Check sheet for the modelled part. Datum: model origin and axes. Units: mm. A direction names the side the tool comes from. Round coordinates to 2 decimals unless told otherwise and drop trailing zeros. Write each loop counter-clockwise with the first axis right and the second up, starting at its lowest first coordinate (ties: lowest second). Pieces come first, ordered by that corner, then holes. Notation, with made-up numbers: (5.5, 30) -> (22.5, 30) arc R28 ccw to (22.5, 66) -> close; hole circle Ø3 at (9, -10.75). An arc over 180 degrees is marked (long way). One line per item, written item: value.
from build123d import *

# Parameters (mm, degrees)
ESQUISSE1_W              = 175
ESQUISSE1_H              = 277
BOSS_EXTRU_2_DEPTH       = 190
ESQUISSE2_W              = 80
ESQUISSE2_H              = 80
ENL_V_MAT_EXTRU_2_DEPTH  = 15
ESQUISSE6_R              = 6.5
BOSS_EXTRU_4_DEPTH       = 15
CHANFREIN2_SIZE          = 1
ENL_V_START              = -10
ESQUISSE12_OUTSIDE_W     = 252.75
ESQUISSE12_OUTSIDE_H     = 354.75
ESQUISSE12_OUTSIDE_W_2   = 155
ESQUISSE12_OUTSIDE_H_2   = 257
ENL_V_MAT_EXTRU_5_DEPTH  = 155
CHANFREIN5_SIZE          = 10
CONG_1_R                 = 5
ENL_V_MAT_EXTRU_10_REACH = 326.86
ESQUISSE13_R             = 2.5
CHANFREIN8_SIZE          = 5
CONG_3_R                 = 10
ESQUISSE14_R             = 10
ESQUISSE14_R_2           = 9
ENL_V_MAT_EXTRU_11_DEPTH = 1
ESQUISSE15_W             = 4
ESQUISSE15_H             = 10
ENL_V_MAT_EXTRU_12_DEPTH = 1


with BuildPart() as part:
    # Esquisse1 → Boss.-Extru.2 (new body)
    with BuildSketch(Plane.XY):
        with Locations((87.5, 138.5)):
            Rectangle(ESQUISSE1_W, ESQUISSE1_H)
    extrude(amount=BOSS_EXTRU_2_DEPTH)

    # Esquisse2 → Enlèv. mat.-Extru.2 (cut)
    with BuildSketch(Plane.XY.offset(190)):
        with Locations((135, 40)):
            Rectangle(ESQUISSE2_W, ESQUISSE2_H)
        with Locations((135, 237)):
            Rectangle(ESQUISSE2_W, ESQUISSE2_H)
    extrude(amount=-ENL_V_MAT_EXTRU_2_DEPTH, mode=Mode.SUBTRACT)

    # Esquisse6 → Boss.-Extru.4 (add)
    with BuildSketch(Plane.XY.offset(175)):
        with Locations((135, 40)):
            Circle(ESQUISSE6_R)
        with Locations(Location((135, 237, 0), (0, 0, 180))):
            Circle(ESQUISSE6_R)
    extrude(amount=BOSS_EXTRU_4_DEPTH)

    # Chanfrein2
    chanfrein2_edges = [part.edges().sort_by_distance(p)[0] for p in [
        (128.5, 40, 190),
        (141.5, 237, 190),
    ]]
    chamfer(chanfrein2_edges, length=CHANFREIN2_SIZE)

    # Esquisse12 outside → Enlèv. mat.-Extru.5 (cut)
    with BuildSketch(Plane(origin=(0, 0, 0), x_dir=(-1, 0, 0), z_dir=(0, 0, -1)).offset(ENL_V_START)):
        with Locations((-87.5, 138.5)):
            Rectangle(ESQUISSE12_OUTSIDE_W, ESQUISSE12_OUTSIDE_H)
        with Locations((-87.5, 138.5)):
            Rectangle(ESQUISSE12_OUTSIDE_W_2, ESQUISSE12_OUTSIDE_H_2, mode=Mode.SUBTRACT)
    extrude(amount=-ENL_V_MAT_EXTRU_5_DEPTH, mode=Mode.SUBTRACT)

    # Chanfrein5
    chanfrein5_edges = [part.edges().sort_by_distance(p)[0] for p in [
        (165, 138.5, 10),
        (87.5, 267, 10),
        (10, 138.5, 10),
        (87.5, 10, 10),
    ]]
    chamfer(chanfrein5_edges, length=CHANFREIN5_SIZE - 0.0001)  # a hair under: the kernel refuses the full size

    # Congé1
    cong_1_edges = [part.edges().sort_by_distance(p)[0] for p in [
        (175, 138.5, 190),
        (135, 80, 190),
        (95, 40, 190),
        (47.5, 277, 190),
        (95, 237, 190),
        (135, 197, 190),
        (0, 138.5, 190),
        (47.5, 0, 190),
    ]]
    fillet(cong_1_edges, radius=CONG_1_R)

    # Esquisse13 → Enlèv. mat.-Extru.10 (cut, up to next)
    with BuildSketch(Plane.XZ.offset(-80), mode=Mode.PRIVATE) as enl_v_mat_extru_10_sk1:
        with Locations((100, 180)):
            Circle(ESQUISSE13_R)
    enl_v_mat_extru_10_tool1 = extrude(enl_v_mat_extru_10_sk1.sketch, amount=-ENL_V_MAT_EXTRU_10_REACH, mode=Mode.PRIVATE) & part.part
    # Esquisse13 → Enlèv. mat.-Extru.10 (cut, up to next)
    with BuildSketch(Plane.XZ.offset(-80), mode=Mode.PRIVATE) as enl_v_mat_extru_10_sk2:
        with BuildLine():
            Line((145, 175), (175, 175))
            Line((175, 175), (175, 190))
            Line((175, 190), (135, 190))
            Line((135, 190), (135, 185))
            ThreePointArc((135, 185), (137.928932188, 177.928932188), (145, 175))
        make_face()
    enl_v_mat_extru_10_tool2 = extrude(enl_v_mat_extru_10_sk2.sketch, amount=-ENL_V_MAT_EXTRU_10_REACH, mode=Mode.PRIVATE) & part.part
    add(enl_v_mat_extru_10_tool1.solids().sort_by_distance((100, 80, 180))[0], mode=Mode.SUBTRACT)
    add(enl_v_mat_extru_10_tool2.solids().sort_by_distance((155.659019, 80, 182.695347))[0], mode=Mode.SUBTRACT)

    # Chanfrein8
    chanfrein8_edges = [part.edges().sort_by_distance(p)[0] for p in [
        (135, 81.464466094, 188.535533906),
        (137.928932188, 80, 177.928932188),
        (137.928932188, 197, 177.928932188),
        (135, 195.535533906, 188.535533906),
        (135, 138.5, 190),
    ]]
    chamfer(chanfrein8_edges, length=CHANFREIN8_SIZE - 0.0001)  # a hair under: the kernel refuses the full size

    # Congé3
    cong_3_edges = [part.edges().sort_by_distance(p)[0] for p in [
        (87.5, 267, 165),
        (165, 138.5, 165),
        (87.5, 10, 165),
        (10, 138.5, 165),
    ]]
    fillet(cong_3_edges, radius=CONG_3_R - 0.0001)  # a hair under: the kernel refuses the full size

    # Esquisse14 → Enlèv. mat.-Extru.11 (cut)
    # profile 1 of 2: a face of its own
    with BuildSketch(Plane.XY.offset(175)):
        with Locations((158.25, 40)):
            Circle(ESQUISSE14_R)
        with Locations((158.25, 40)):
            Circle(ESQUISSE14_R_2, mode=Mode.SUBTRACT)
    # profile 2 of 2: a face of its own
    with BuildSketch(Plane.XY.offset(175)):
        with Locations(Location((158.25, 237, 0), (0, 0, 180))):
            Circle(ESQUISSE14_R)
        with Locations(Location((158.25, 237, 0), (0, 0, 180))):
            Circle(ESQUISSE14_R_2, mode=Mode.SUBTRACT)
    extrude(amount=-ENL_V_MAT_EXTRU_11_DEPTH, mode=Mode.SUBTRACT)

    # Esquisse15 → Enlèv. mat.-Extru.12 (cut)
    with BuildSketch(Plane.XY.offset(175)):
        with Locations((158.25, 40)):
            Rectangle(ESQUISSE15_W, ESQUISSE15_H)
        Polygon((156.583333333, 235.333333333), (153.25, 235.333333333), (153.25, 238.666666667), (156.583333333, 238.666666667), (156.583333333, 242), (159.916666667, 242), (159.916666667, 238.666666667), (163.25, 238.666666667), (163.25, 235.333333333), (159.916666667, 235.333333333), (159.916666667, 232), (156.583333333, 232), align=None)
    extrude(amount=-ENL_V_MAT_EXTRU_12_DEPTH, mode=Mode.SUBTRACT)


solid = part.part
Item 1: Release check for a two-part mould opening along X. For faces 4 (the cylindrical face through (165.39, 242.48, 174.51)), 5 (the flat face through (86, 140, 0)), 6 (the cylindrical face through (6.99, 140.44, 162.15)) record: pulls with the +X half, pulls with the -X half, needs draft (parallel to the pull), parting line crosses it, or undercut.
Result set:
face 4: undercut
face 5: needs draft
face 6: pulls with the -X half
Item 2: Material ranges on line 1 along X through (y, z) = (237, 174.6); line 2 along Z through (x, y) = (100, 155); line 3 along Y through (x, z) = (40, 50.5), recorded low to high.
Result set:
line 1: 0 to 148.25, 149.25 to 153.25, 163.25 to 167.25, 168.25 to 175
line 2: 0 to 177.5, 182.5 to 190
line 3: 10 to 267
Item 3: Depth check by flat-ended pin: pin 1 (14.5 mm diameter, centred on x = 161.5, y = 240, fed in from +Z); pin 2 (4 mm diameter, centred on x = 77, z = 69.5, fed in from -Y); pin 3 (5 mm diameter, centred on y = 38, z = 180, fed in from +X). Enter the tip coordinate at first touch or a pass-through.
Result set:
pin 1: z = 175
pin 2: y = 10
pin 3: x = 141.5
Item 4: Sectioned sample at D-D (z = 131). Enter the section's corners in (x, y).
Result set:
outline: (10, 10) -> (165, 10) -> (165, 267) -> (10, 267) -> close
Item 5: Tool access check on faces 1 (the flat face through (170, 137, 15)), 2 (the flat face through (89, 5, 15)), 3 (the flat face through (89, 272, 15)). Record the directions out of +Z, -Z, +X, -X, +Y, -Y that give a thin tool (end or side, any length) a straight path to the whole face; none if there is none.
Result set:
face 1: +X, +Y, -Y
face 2: +X, -X, -Y
face 3: +X, -X, +Y
